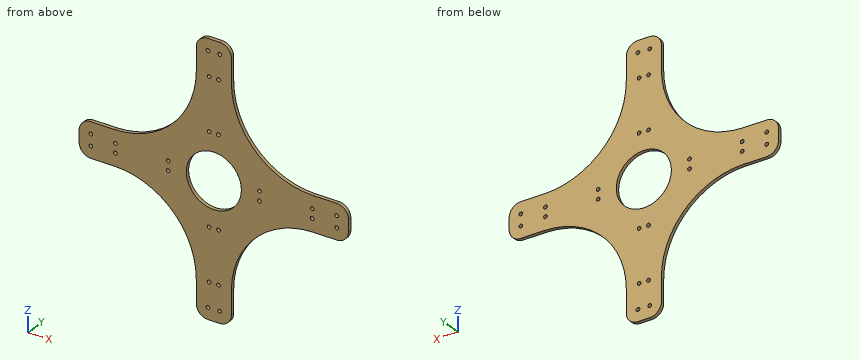
```python
from build123d import *

# Parameters (mm, degrees)
BOSS_EXTRUDE1_DEPTH      = 1.5
M3_CLEARANCE_HOLE1_D     = 3.2
M3_CLEARANCE_HOLE1_DEPTH = 3
SKETCH5_R                = 23.5
CUT_EXTRUDE1_DEPTH       = 1
CUT_EXTRUDE1_DEPTH_BACK  = 4
SKETCH7_R                = 1.6
CUT_EXTRUDE2_DEPTH       = 4


with BuildPart() as part:
    # Sketch1 → Boss-Extrude1 (new body, symmetric)
    with BuildSketch(Plane(origin=(0, 0, 0), x_dir=(1, 0, 0), z_dir=(0, 1, 0))):
        with BuildLine():
            Line((85, 15), (105, 15))
            ThreePointArc((105, 15), (112.071067812, 12.071067812), (115, 5))
            Line((115, 5), (115, -5))
            ThreePointArc((115, -5), (112.071067812, -12.071067812), (105, -15))
            Line((105, -15), (85, -15))
            ThreePointArc((85, -15), (35.502525317, -35.502525317), (15, -85))
            Line((15, -85), (15, -105))
            ThreePointArc((15, -105), (12.071067812, -112.071067812), (5, -115))
            Line((5, -115), (-5, -115))
            ThreePointArc((-5, -115), (-12.071067812, -112.071067812), (-15, -105))
            Line((-15, -105), (-15, -85))
            ThreePointArc((-15, -85), (-35.502525317, -35.502525317), (-85, -15))
            Line((-85, -15), (-105, -15))
            ThreePointArc((-105, -15), (-112.071067812, -12.071067812), (-115, -5))
            Line((-115, -5), (-115, 5))
            ThreePointArc((-115, 5), (-112.071067812, 12.071067812), (-105, 15))
            Line((-105, 15), (-85, 15))
            ThreePointArc((-85, 15), (-35.502525317, 35.502525317), (-15, 85))
            Line((-15, 85), (-15, 105))
            ThreePointArc((-15, 105), (-12.071067812, 112.071067812), (-5, 115))
            Line((-5, 115), (5, 115))
            ThreePointArc((5, 115), (12.071067812, 112.071067812), (15, 105))
            Line((15, 105), (15, 85))
            ThreePointArc((15, 85), (35.502525317, 35.502525317), (85, 15))
        make_face()
    extrude(amount=BOSS_EXTRUDE1_DEPTH, both=True)

    # M3 Clearance Hole1
    with Locations(Plane(origin=(0, 1.5, 0), x_dir=(1, 0, 0), z_dir=(0, 1, 0))):
        with Locations((-105, 5), (-105, -5), (-5, 105), (5, 105), (105, 5), (105, -5), (5, -105), (-5, -105)):
            Hole(M3_CLEARANCE_HOLE1_D / 2, depth=M3_CLEARANCE_HOLE1_DEPTH)

    # Sketch5 → Cut-Extrude1 (cut, two sides)
    with BuildSketch(Plane(origin=(0, 1.5, 0), x_dir=(1, 0, 0), z_dir=(0, 1, 0))) as cut_extrude1_sk:
        Circle(SKETCH5_R)
    extrude(amount=CUT_EXTRUDE1_DEPTH, mode=Mode.SUBTRACT)
    extrude(cut_extrude1_sk.sketch, amount=-CUT_EXTRUDE1_DEPTH_BACK, mode=Mode.SUBTRACT)

    # Sketch7 → Cut-Extrude2 (cut, through all)
    with BuildSketch(Plane.XZ.offset(1.5)):
        with Locations((39, 4)):
            Circle(SKETCH7_R)
        with Locations((39, -4)):
            Circle(SKETCH7_R)
        with Locations((84, 4)):
            Circle(SKETCH7_R)
        with Locations((84, -4)):
            Circle(SKETCH7_R)
        with Locations((-4, -39)):
            Circle(SKETCH7_R)
        with Locations((4, -39)):
            Circle(SKETCH7_R)
        with Locations((4, -84)):
            Circle(SKETCH7_R)
        with Locations((-4, -84)):
            Circle(SKETCH7_R)
        with Locations((-39, 4)):
            Circle(SKETCH7_R)
        with Locations((-39, -4)):
            Circle(SKETCH7_R)
        with Locations((-84, -4)):
            Circle(SKETCH7_R)
        with Locations((-84, 4)):
            Circle(SKETCH7_R)
        with Locations((4, 39)):
            Circle(SKETCH7_R)
        with Locations((-4, 39)):
            Circle(SKETCH7_R)
        with Locations((-4, 84)):
            Circle(SKETCH7_R)
        with Locations((4, 84)):
            Circle(SKETCH7_R)
    extrude(amount=-CUT_EXTRUDE2_DEPTH, mode=Mode.SUBTRACT)


solid = part.part
```
Here's how the part is built. I have some questions about the finished solid (model axes, mm). Coordinates: 2 decimals unless noted, no trailing zeros. Order: outer loops, then holes, each group sorted by start corner. A loop starts at its lowest first (then second) coordinate and runs counter-clockwise, first axis right, second up.
1) Imagine slicing it at A-A on x = -97. List the corners of the cut face in (y, z) for me, and give its area (3 significant figures).
2) Will these pins go through, and if not, where does the flat tip stop? pin 1 (2.5 mm diameter, centred on x = 5, z = 105, fed in from +Y); pin 2 (1.5 mm diameter, centred on x = 13.5, y = -0.5, fed in from +Z); pin 3 (1.5 mm diameter, centred on x = 98.5, y = 0, fed in from -Z); pin 4 (1 mm diameter, centred on y = 1, z = 50.5, fed in from +X).
3) Imagine slicing it at C-C on z = -29. List the corners of the cut face in (x, y) for me.
4) I need wall thicknesses on line 1 (Z direction, x = 105, y = 0.5); line 2 (Z direction, x = -84, y = -0.5). Which ranges of each line are inside material? Lowest first, please.
5) Imagine slicing it at B-B on y = 0.25. State how many separate pieces and enclosed holes the cut face has, and give its area (3 significant figures).
Response values:
1. outline: (-1.5, -15) - (1.5, -15) - (1.5, 15) - (-1.5, 15) - close
1. area: 90.0 mm2
2. pin 1: passes through
2. pin 2: stops at z = 111.32
2. pin 3: stops at z = -15
2. pin 4: stops at x = 24.38
3. outline: (-43, -1.5) - (43, -1.5) - (43, 1.5) - (-43, 1.5) - close
4. line 1: z = -15 to -6.6, -3.4 to 3.4, 6.6 to 15
4. line 2: z = -15.01 to -5.6, -2.4 to 2.4, 5.6 to 15.01
5. separate pieces: 1
5. enclosed holes: 25
5. area: 15,000 mm2
